Autodesk Inventor part; units mm, degrees
ref_plane "Plano inicial" through (0, 0, 0) normal (0, 0, 1) x (1, 0, 0)
ref_plane "Plano final" through (0, 0, 225) normal (0, 0, 1) x (1, 0, 0)
ref_plane "Plano de trabalho7" through (0, -25, 225) normal (0, 0.7071, 0.7071) x (1, 0, 0)
ref_plane "Plano inicial" through (0, 0, 0) normal (0, 0, 1) x (1, 0, 0)
ref_plane "Plano final" through (0, 0, 225) normal (0, 0, 1) x (1, 0, 0)
sketch "Esboço" plane through (0, 0, 0) normal (0, 0, 1) x (1, 0, 0)
  line L0 (-15, -21.25) -> (-15, 21.25)
  line L1 (-11.25, 25) -> (11.25, 25)
  line L2 (15, 21.25) -> (15, -21.25)
  line L3 (11.25, -25) -> (-11.25, -25)
  arc A0 (-15, -21.25) -> (-11.25, -25) centre (-11.25, -21.25) ccw
  arc A1 (-11.25, 25) -> (-15, 21.25) centre (-11.25, 21.25) ccw
  arc A2 (15, 21.25) -> (11.25, 25) centre (11.25, 21.25) ccw
  arc A3 (11.25, -25) -> (15, -21.25) centre (11.25, -21.25) ccw
  arc A4 (-11.25, 22.5) -> (-12.5, 21.25) centre (-11.25, 21.25) ccw
  line L4 (-11.25, 22.5) -> (11.25, 22.5)
  arc A5 (12.5, 21.25) -> (11.25, 22.5) centre (11.25, 21.25) ccw
  line L5 (12.5, 21.25) -> (12.5, -21.25)
  arc A6 (11.25, -22.5) -> (12.5, -21.25) centre (11.25, -21.25) ccw
  line L6 (11.25, -22.5) -> (-11.25, -22.5)
  arc A7 (-12.5, -21.25) -> (-11.25, -22.5) centre (-11.25, -21.25) ccw
  line L7 (-12.5, -21.25) -> (-12.5, 21.25)
  line L8 (0, 36.0873) -> (0, -36.0873) construction
  line L9 (-22.0873, 0) -> (22.0873, 0) construction
  dimension "d7" = 3.75
  dimension "d10" = 50
  dimension "d11" = 30
  dimension "d12" = 2.5
  dimension "d15" = 25
  dimension "d16" = 15
extrude "Corpo" add sketch "Esboço" along normal up to surface (225 mm away) from surface at 0
sketch "Sketch3" plane through (0, 0, 0) normal (0, 0, 1) x (1, 0, 0)
  line L0 (0, 0) -> (10, 0)
ref_plane "Work Plane3" through (0, 0, 0) normal (0, -1, 0) x (1, 0, 0)
sketch "Sketch4" plane through (0, 0, 0) normal (0, -1, 0) x (1, 0, 0)
  line L0 (-2, 0) -> (12, 0)
  line L1 (-2, 225) -> (12, 225)
  dimension "d18" = 225
ref_plane "Plano de trabalho7" through (0, -25, 225) normal (0, 0.7071, 0.7071) x (1, 0, 0)
split "Dividir4" plane through (0, -25, 225) removes the side toward (0, 0.7071, 0.7071)
ref_plane "Plano de trabalho9" through (15, 0, 0) normal (-0.7071, 0, -0.7071) x (-0.7071, 0, 0.7071)
split "Dividir6" plane through (15, 0, 0) removes the side toward (-0.7071, 0, -0.7071)
equation "\"d7\" = G_IR"
equation "\"d10\" = G_H"
equation "\"d11\" = G_W"
equation "\"d12\" = G_T"
equation "\"d15\" = 0.5 * d10"
equation "\"d16\" = 0.5 * d11"
equation "\"d3\" = G_L"
equation "\"G_W\" = 30"
equation "\"G_H\" = 50"
equation "\"G_T\" = 2.5"
equation "\"G_IR\" = 3.75"
equation "\"G_L\" = d18"
equation "\"G_OFFSET_START\" = 0"
equation "\"d14\" = G_OFFSET_END + B_L"
equation "\"B_L\" = 175"
properties part number "ISO 12633-2 - 50x30x2.5 - 225" material "Aço, suave"
Input: part model. Units: mm. Frame: model coordinates. A direction names the side the tool comes from. Round coordinates to 2 decimals unless told otherwise and drop trailing zeros. Loops run counter-clockwise (first coordinate to the right, second up) from the corner with the lowest first, then second, coordinate; pieces in that order, holes last. Notation, with made-up numbers: (-35, -19.5) -> (-22, -19.5) arc R29 ccw to (-22, 16.5) -> close; hole circle Ø10 at (0.5, 45.25). An arc over 180 degrees is marked (long way). Answer as a JSON object with one key per item and string values. Group by question number.
1) Section query B-B on x = -4.5. Output: boundary loops of the cut face in (y, z), plus the area to 4 significant figures.
2) Section query A-A on y = -3. Output: boundary loops of the cut face in (x, z), plus the area to 3 significant figures.
3) Draft query along Y for faces 3 (the cylindrical face through (13.931, -23.872, 110.925)), 4 (the flat face through (-15, 0, 124)), 5 (the flat face through (-12.5, 0, 123)). Return one class per face: +Y half, -Y half, draft (parallel to the pull), parting line (faces both ways), or undercut.
4) Reachability of faces 1 (the flat face through (0, -22.5, 112)), 2 (the flat face through (0, 25, 88)) from +Z, -Z, +X, -X, +Y, -Y: full face, straight path, thin tool, end or side. Return the list, or none.
5) Ray query, L1, parallel to Y at x = 3, z = 13; L2, parallel to X at y = -12.5, z = 210; L3, parallel to Y at x = -11, z = 200.5. Return the intervals inside material, ascending.
6) Section query D-D on z = 50.5. Output: boundary loops of the cut face in (x, y), plus the area to 3 significant figures.
7) Section query C-C on z = 200.5. Output: boundary loops of the cut face in (x, y).
Reply:
{
 "1": {"outline": "(-25, 19.5) -> (-22.5, 19.5) -> (-22.5, 222.5) -> (-25, 225) -> close; (22.5, 19.5) -> (25, 19.5) -> (25, 175) -> (22.5, 177.5) -> close", "area": "902.5 mm2"},
 "2": {"outline": "(-15, 30) -> (-12.5, 27.5) -> (-12.5, 203) -> (-15, 203) -> close; (12.5, 2.5) -> (15, 0) -> (15, 203) -> (12.5, 203) -> close", "area": "940 mm2"},
 "3": {"face 3": "-Y half", "face 4": "draft", "face 5": "undercut"},
 "4": {"face 1": "+Z, -Z", "face 2": "+Z, -Z, +X, -X, +Y"},
 "5": {"L1": "y = -25 to -22.5, 22.5 to 25", "L2": "x = -15 to -12.5, 12.5 to 15", "L3": "y = -25 to -22.5"},
 "6": {"outline": "(-15, -21.25) arc R3.75 ccw to (-11.25, -25) -> (11.25, -25) arc R3.75 ccw to (15, -21.25) -> (15, 21.25) arc R3.75 ccw to (11.25, 25) -> (-11.25, 25) arc R3.75 ccw to (-15, 21.25) -> close; hole (-12.5, -21.25) arc R1.25 ccw to (-11.25, -22.5) -> (11.25, -22.5) arc R1.25 ccw to (12.5, -21.25) -> (12.5, 21.25) arc R1.25 ccw to (11.25, 22.5) -> (-11.25, 22.5) arc R1.25 ccw to (-12.5, 21.25) -> close", "area": "364 mm2"},
 "7": {"outline": "(-15, -21.25) arc R3.75 ccw to (-11.25, -25) -> (11.25, -25) arc R3.75 ccw to (15, -21.25) -> (15, -0.5) -> (12.5, -0.5) -> (12.5, -21.25) arc R1.25 cw to (11.25, -22.5) -> (-11.25, -22.5) arc R1.25 cw to (-12.5, -21.25) -> (-12.5, -0.5) -> (-15, -0.5) -> close"}
}
